```python
from build123d import *

# Parameters (mm, degrees)
FILLET1_R           = 5
FILLET2_R           = 3
BOSS_EXTRUDE1_DEPTH = 25
CUT_EXTRUDE3_START  = -5
SKETCH24_R          = 10
CUT_EXTRUDE3_DEPTH  = 21


with BuildPart() as part:
    # Sketch2 → Revolve1 (revolve)
    with BuildSketch(Plane(origin=(0, 0, 0), x_dir=(0, 0, -1), z_dir=(1, 0, 0))):
        Polygon((-185, -25), (-205, -25), (-205, 10), (-185, 10), (-185, 5), (-190, 5), (-190, 0), (-185, 0), align=None)
    revolve(axis=Axis((0, 0, 0), (0, 1, 0)))

    # Fillet1
    fillet1_edges = [part.edges().sort_by_distance(p)[0] for p in [
        (0, 10, -205),
    ]]
    fillet(fillet1_edges, radius=FILLET1_R)

    # Fillet2
    fillet2_edges = [part.edges().sort_by_distance(p)[0] for p in [
        (0, 10, -185),
    ]]
    fillet(fillet2_edges, radius=FILLET2_R)

    # Sketch15 → Boss-Extrude1 (add)
    with BuildSketch(Plane(origin=(0, 0, 0), x_dir=(1, 0, 0), z_dir=(0, 1, 0))):
        with BuildLine():
            ThreePointArc((-118.887266817, 141.742081926), (-66.69307667, 151.357832715), (-24.375030373, 183.387180289))
            ThreePointArc((-24.375030373, 183.387180289), (-74.596246578, 169.293827402), (-118.887266817, 141.742081926))
        make_face()
        with BuildLine():
            ThreePointArc((-118.944143978, -141.694356321), (-137.477235911, -91.962870803), (-176.368437347, -55.849568556))
            ThreePointArc((-176.368437347, -55.849568556), (-153.768371484, -102.860526594), (-118.944143978, -141.694356321))
        make_face()
    extrude(amount=-BOSS_EXTRUDE1_DEPTH)

    # Sketch24 → Cut-Extrude3 (cut, through all)
    with BuildSketch(Plane(origin=(0, 0, 0), x_dir=(1, 0, 0), z_dir=(0, 1, 0)).offset(CUT_EXTRUDE3_START)):
        with Locations((-74.596246578, 169.293827402)):
            Circle(SKETCH24_R)
        with Locations((-153.768371484, -102.860526594)):
            Circle(SKETCH24_R)
    extrude(amount=-CUT_EXTRUDE3_DEPTH, mode=Mode.SUBTRACT)


solid = part.part
```
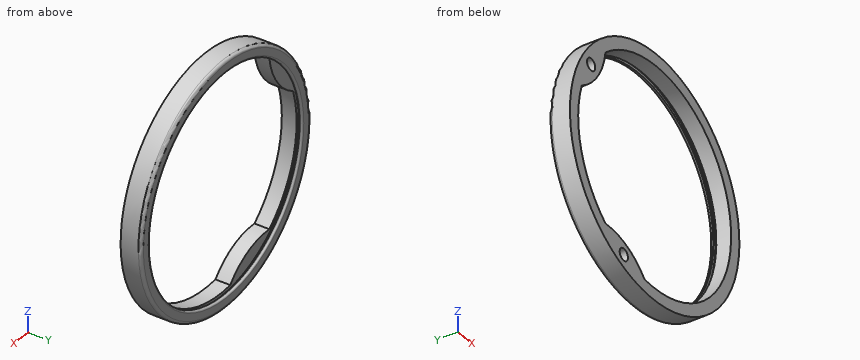
Check sheet for the modelled part. Datum: model origin and axes. Units: mm. Give positions to 0.01 mm unless a question says otherwise; leave off trailing zeros. Write each loop counter-clockwise with the first axis right and the second up, starting at its lowest first coordinate (ties: lowest second). Pieces come first, ordered by that corner, then holes. Notation, with made-up numbers: (44.5, -37) - (98.5, -37) arc R17 ccw to (98.5, -6) - close; hole circle Ø7 at (0, 51). An arc over 180 degrees is marked (long way). Answer as a JSON object with one key per item and string values. Group by question number.
1) Sectioned sample at C-C (y = -15). Record the cut outline in (x, z).
2) Sectioned sample at B-B (x = 0). Record the cut outline in (y, z), then the cut area to 3 significant figures.
3) Sectioned sample at A-A (z = 0). Record the cut outline in (x, y), then the cut area to 3 significant figures.
4) Depth check by flat-ended pin: P1, Ø2, axis at y = -15, z = -137.5, coming from the +X side; P2, Ø3, axis at x = -129, y = -5.5, coming from the -Z side; P3, Ø5, axis at y = 5.5, z = 77.5, coming from the +X side. Enter the tip coordinate at first touch or a pass-through.
5) Thickness scan on probe 1 along Z at (x, y) = (-162, -13.5); probe 2 along X at (y, z) = (3, 0); probe 3 along X at (y, z) = (-14.5, -63.5). Record the ranges inside material, lowest first. Write a range as from..to.
Geometry results:
{
 "1": {"outline": "circle Ø410 at (0, 0); hole (-176.37, 55.85) arc R185 ccw to (-118.89, -141.74) arc R115 cw to (-24.38, -183.39) arc R185 ccw (long way) to (-118.94, 141.69) arc R115 cw to start; hole circle Ø20 at (-153.77, 102.86); hole circle Ø20 at (-74.6, -169.29)"},
 "2": {"outline": "(-25, -205) - (5, -205) arc R5 ccw to (10, -200) - (10, -188) arc R3 ccw to (7, -185) - (5, -185) - (5, -190) - (0, -190) - (0, -185) - (-25, -185) - close; (-25, 185) - (0, 185) - (0, 190) - (5, 190) - (5, 185) - (7, 185) arc R3 ccw to (10, 188) - (10, 200) arc R5 ccw to (5, 205) - (-25, 205) - close", "area": "1,340 mm^2"},
 "3": {"outline": "(-205, -25) - (-185, -25) - (-185, 0) - (-190, 0) - (-190, 5) - (-185, 5) - (-185, 7) arc R3 ccw to (-188, 10) - (-200, 10) arc R5 ccw to (-205, 5) - close; (185, -25) - (205, -25) - (205, 5) arc R5 ccw to (200, 10) - (188, 10) arc R3 ccw to (185, 7) - (185, 5) - (190, 5) - (190, 0) - (185, 0) - close", "area": "1,340 mm^2"},
 "4": {"P1": "stops at x = 152.95", "P2": "stops at z = -160.53", "P3": "stops at x = 190.78"},
 "5": {"probe 1": "z = -125.62..-89.34, 65.49..97.18, 108.54..125.62", "probe 2": "x = -205..-190, 190..205", "probe 3": "x = -194.92..-173.76, 173.76..194.92"}
}
